Can you work these out from the model? Positions are in its coordinate system, mm. Give positions to 0.01 mm unless a question says otherwise; leave off trailing zeros. Order: outer loops, then holes, each group sorted by start corner. A loop starts at its lowest first (then second) coordinate and runs counter-clockwise, first axis right, second up.
```python
from build123d import *

# Parameters (mm, degrees)
BOSS_EXTRUDE1_DEPTH = 3
CUT_EXTRUDE1_DEPTH  = 123


with BuildPart() as part:
    # Sketch1 → Boss-Extrude1 (new body)
    with BuildSketch(Plane.XY):
        with BuildLine():
            Line((0, 61), (-130, 61))
            Line((-130, 61), (-130, -61))
            Line((-130, -61), (0, -61))
            ThreePointArc((0, -61), (-61, 0), (0, 61))
        make_face()
    extrude(amount=BOSS_EXTRUDE1_DEPTH)

    # Sketch3 → Cut-Extrude1 (cut)
    with BuildSketch(Plane(origin=(0, -61, 0), x_dir=(-1, 0, 0), z_dir=(0, -1, 0))):
        Polygon((130, -3), (60, 0), (130, 0), align=None)
    extrude(amount=-CUT_EXTRUDE1_DEPTH, mode=Mode.SUBTRACT)


solid = part.part
```
1) Suppose I cut it at D-D (y = 0). Please give me the cut outline in (x, z), and give its area (3 significant figures).
2) We'd pull the mould along X, two halves only. Please class faces 1 (the face through (-46, 49, 0)), 2 (the face through (-60.985, -1.341, 1.479)), 3 (the face through (-95.49, -0.85, 1.52)): +X half, -X half, draft (parallel to the pull), parting line (faces both ways), or undercut.
3) Suppose I cut it at C-C (y = 14). Please give me the cut outline in (x, z).
4) Suppose I cut it at A-A (x = -30.5). Please give me the cut outline in (y, z).
5) Suppose I cut it at B-B (z = 1.5). Please give me the cut outline in (x, y).
6) I'm going to push a flat-ended pin straight in: pin 1 Ø3 at (x, y) = (-82, 13) entering from -Z. Where does the tip first touch, or does it pass through?
7) If I drill on line 1 (Y direction, x = -48.5, z = 1.4); line 2 (Y direction, x = -29, z = 2.4); line 3 (Z direction, x = -117, y = -1), over which ranges is the centre line in solid material (lowest first)?
Results:
1. outline: (-130, 3) - (-61, 0.04) - (-61, 3) - close
1. area: 102 mm2
2. face 1: draft
2. face 2: +X half
2. face 3: -X half
3. outline: (-130, 3) - (-60, 0) - (-59.37, 0) - (-59.37, 3) - close
4. outline: (-61, 0) - (-52.83, 0) - (-52.83, 3) - (-61, 3) - close; (52.83, 0) - (61, 0) - (61, 3) - (52.83, 3) - close
5. outline: (-95, -61) - (0, -61) arc R61 cw to (0, 61) - (-95, 61) - close
6. pin 1: stops at z = 0.88
7. line 1: y = -61 to -37, 37 to 61
7. line 2: y = -61 to -53.67, 53.67 to 61
7. line 3: z = 2.44 to 3
